from build123d import *

# Parameters (mm, degrees)
F1_DEPTH = 15
F3_DEPTH = 5
F4_R     = 13


with BuildPart() as f1:
    # F0 (on Front) → F1 (new body)
    with BuildSketch(Plane.XZ):
        with BuildLine():
            ThreePointArc((25, 7), (21.192388, 16.192388), (12, 20))
            Line((12, 20), (-12, 20))
            ThreePointArc((-12, 20), (-21.192388, 16.192388), (-25, 7))
            Line((-25, 7), (-25, -7))
            ThreePointArc((-25, -7), (-21.192388, -16.192388), (-12, -20))
            Line((-12, -20), (12, -20))
            ThreePointArc((12, -20), (21.192388, -16.192388), (25, -7))
            Line((25, -7), (25, 7))
        make_face()
    extrude(amount=-F1_DEPTH)

    # F2 (on Top) → F3 (join, symmetric)
    with BuildSketch(Plane.XY):
        with BuildLine():
            Line((-25, -25), (-8, -25))
            ThreePointArc((-8, -25), (0, -17), (8, -25))
            Line((8, -25), (25, -25))
            Line((25, -25), (25, 0))
            Line((25, 0), (-25, 0))
            Line((-25, 0), (-25, -25))
        make_face()
    extrude(amount=F3_DEPTH, both=True)

    # F4
    f4_edges = [f1.edges().sort_by_distance(p)[0] for p in [
        (0, 0, 5),
        (0, 0, -5),
    ]]
    fillet(f4_edges, radius=F4_R)


solid = f1.part
Source: CAD feature listing. Evaluate the final solid. Frame: model axes, mm. A direction names the side the tool comes from. Give positions to 0.01 mm unless a question says otherwise; leave off trailing zeros. Write each loop counter-clockwise with the first axis right and the second up, starting at its lowest first coordinate (ties: lowest second). Pieces come first, ordered by that corner, then holes. Notation, with made-up numbers: M 12.25,18.5 L 50.25,18.5 A8 ccw 50.25,25.5 Z; hole C -33.75,-22.5 d8. An arc over 180 degrees is marked long. Return JSON: item names as keys, results as strings. Group by question number.
1) Ray query, L1, parallel to Z at x = 18, y = -20; L2, parallel to Y at x = 16.5, z = -18; L3, parallel to Y at x = -11, z = 8.5. Return the intervals inside material, ascending.
2) Cut plane D-D, the plane z = 4. Output: boundary loops of the cut face in (x, y).
3) Draft query along X for faces 4 (the face through (0, 0, 19)), 5 (the face through (21.091, 6.658, -16.293)), 6 (the face through (-25, -5, 0)), 7 (the face through (0, -17, 0)). Return one class per face: released by +X, released by -X, zero draft, split by the parting line, or undercut.
4) Cut plane A-A, the plane y = -20. Output: boundary loops of the cut face in (x, z) (3 decimals), then the cut area to 3 significant figures.
5) Cut plane C-C, the plane y = 5. Output: boundary loops of the cut face in (x, z).
6) First-contact query: pin 1 Ø2 at (x, z) = (7, 19.5) entering from -Y; pin 2 Ø10 at (x, y) = (3, -12) entering from -Z; pin 3 Ø13 at (x, y) = (9.5, -18.5) entering from -Z; pin 4 Ø3.5 at (x, y) = (-2, -19.5) entering from +Z. Flat tips, straight axial feed; report the tip coordinate or a pass-through.
7) Cut plane B-B, the plane x = 0. Output: boundary loops of the cut face in (y, z), then the cut area to 3 significant figures.
8) Set-up query: faces 1 (the face through (0, -16, 5)), 2 (the face through (0, -16, -5)), 3 (the face through (21.293, 6.658, 16.091)). Return all of +Z, -Z, +X, -X, +Y, -Y with unobstructed straight access to the full face (end or side cutting, diameter ignored); none if empty.
Data:
{
 "1": {"L1": "z = -5 to 5", "L2": "y = 0 to 15", "L3": "y = -4.13 to 15"},
 "2": {"outline": "M -25,-25 L -8,-25 A8 cw 8,-25 L 25,-25 L 25,15 L -25,15 Z"},
 "3": {"face 4": "zero draft", "face 5": "released by +X", "face 6": "released by -X", "face 7": "undercut"},
 "4": {"outline": "M -25,-5 L -6.245,-5 L -6.245,5 L -25,5 Z; M 6.245,-5 L 25,-5 L 25,5 L 6.245,5 Z", "area": "375 mm²"},
 "5": {"outline": "M -25,-7 A13 ccw -12,-20 L 12,-20 A13 ccw 25,-7 L 25,7 A13 ccw 12,20 L -12,20 A13 ccw -25,7 Z"},
 "6": {"pin 1": "stops at y = 0", "pin 2": "stops at z = -6.47", "pin 3": "stops at z = -5.04", "pin 4": "passes through"},
 "7": {"outline": "M -17,-5 L -13,-5 A13 cw 0,-18 L 0,-20 L 15,-20 L 15,20 L 0,20 L 0,18 A13 cw -13,5 L -17,5 Z", "area": "843 mm²"},
 "8": {"face 1": "+Z, +X, -X, -Y", "face 2": "-Z, +X, -X, -Y", "face 3": "+Z, +X, +Y, -Y"}
}
